```python
from build123d import *

# Parameters (mm, degrees)
F0_R     = 24.4478628748
F1_DEPTH = 5
F2_R     = 19.1271532248
F3_DEPTH = 5
F4_W     = 6.9555565715
F4_H     = 47.9025412351
F5_DEPTH = 5
F6_DEPTH = 7


with BuildPart() as f1:
    # F0 (on Top) → F1 (new body)
    with BuildSketch(Plane.XY):
        Circle(F0_R)
    extrude(amount=F1_DEPTH)

    # F2 (on Front) → F3 (cut)
    with BuildSketch(Plane.XZ):
        Circle(F2_R)
    extrude(amount=-F3_DEPTH, mode=Mode.SUBTRACT)

    # F4 (on Top) → F5 (join)
    with BuildSketch(Plane.XY):
        with Locations((24.5456583798, 0.5576470867)):
            Rectangle(F4_W, F4_H)
    extrude(amount=F5_DEPTH)

    # F6 (add): a face of the model
    f6_faces = [f1.faces().sort_by_distance(p)[0] for p in [
        (3.5064630649, -0.1400049466, 5),
    ]]
    extrude(f6_faces, amount=F6_DEPTH)


solid = f1.part
```
Model file for the job. Use its own axes, mm. A direction names the side the tool comes from. Round coordinates to 2 decimals unless told otherwise and drop trailing zeros. Order: outer loops, then holes, each group sorted by start corner. A loop starts at its lowest first (then second) coordinate and runs counter-clockwise, first axis right, second up. Notation, with made-up numbers: (49, 33) -> (108, 33) arc R24 ccw to (108, 55) -> close; hole circle Ø7 at (42, 88.5). An arc over 180 degrees is marked (long way). Use one line per item in the form item = value.
Item 1: Cut at D-D, the plane x = -7.5. Write the cut outline in (y, z), and give its area (3 significant figures).
Returned:
outline = (-23.27, 0) -> (0, 0) -> (0, 12) -> (-23.27, 12) -> close; (5, 0) -> (23.27, 0) -> (23.27, 12) -> (5, 12) -> close
area = 498 mm^2
Item 2: Drill centre lines: line 1 (Y direction, x = 0.5, z = 11.5); line 2 (Y direction, x = 4.5, z = 4.75); line 3 (X direction, y = -17.5, z = 1). Where is each one in solid material? Low to high.
Returned:
line_1 = -24.44 to 0, 5 to 24.44
line_2 = -24.03 to 0, 5 to 24.03
line_3 = -17.07 to 17.07, 21.07 to 28.02
Item 3: Cut at A-A, the plane x = 0. Write the cut outline in (y, z).
Returned:
outline = (-24.45, 0) -> (0, 0) -> (0, 12) -> (-24.45, 12) -> close; (5, 0) -> (24.45, 0) -> (24.45, 12) -> (5, 12) -> close
Item 4: Pull direction X, two halves, no side cores. Call faces 5 (the face through (-18.462, 3, 8)), 6 (the face through (24, 24.509, 6)), 7 (the face through (28.023, 0, 6)): released by +X, released by -X, zero draft, split by the parting line, or undercut.
Returned:
face_5 = undercut
face_6 = zero draft
face_7 = released by +X
Item 5: Cut at C-C, the plane y = 2. Write the cut outline in (x, z), and give its area (3 significant figures).
Returned:
outline = (-24.37, 0) -> (-19.13, 0) arc R19.13 cw to (-18.46, 5) -> (-18.46, 12) -> (-24.37, 12) -> close; (18.46, 5) arc R19.13 cw to (19.13, 0) -> (28.02, 0) -> (28.02, 12) -> (18.46, 12) -> close
area = 181 mm^2
Item 6: Flat gauge pins, fed straight in: pin 1 Ø3.5 at (x, z) = (-5, 4) entering from -Y; pin 2 Ø2 at (x, z) = (13.5, 8) entering from -Y; pin 3 Ø1.5 at (x, z) = (14, 3) entering from +Y; pin 4 Ø8 at (x, y) = (-1, 0.5) entering from -Z. Where does each tip first touch, or does it go through?
Returned:
pin_1 = -24.23
pin_2 = -21.01
pin_3 = 20.55
pin_4 = 0
Item 7: Cut at B-B, the plane z = 8.5. Write the cut outline in (x, y), and give its area (3 significant figures).
Returned:
outline = (21.07, -23.39) -> (28.02, -23.39) -> (28.02, 24.51) -> (21.07, 24.51) -> (21.07, 12.4) arc R24.45 ccw (long way) to (21.07, -12.4) -> close; hole (-18.46, 0) -> (18.46, 0) -> (18.46, 5) -> (-18.46, 5) -> close
area = 1,970 mm^2
Item 8: Tool access for faces 1 (the face through (21.068, -18, 6)), 2 (the face through (21.068, 18, 6)), 3 (the face through (-18.955, 2.465, 2.557)), 4 (the face through (24, -23.394, 6)): list every direction of +Z, -Z, +X, -X, +Y, -Y with a clear straight run to the whole face (end or side of a thin tool).
Returned:
face_1 = +Z, -Z, -Y
face_2 = +Z, -Z, +Y
face_3 = -Z
face_4 = +Z, -Z, +X, -Y
